Can you work these out from the drawing? Everything is in mm from the part's minimum corner. A direction names the side the tool comes from. Give positions to 0.01 mm unless a question says otherwise; leave off trailing zeros. Loops run counter-clockwise (first coordinate to the right, second up) from the corner with the lowest first, then second, coordinate; pieces in that order, holes last. Notation, with made-up numbers: (53.25, 87.5) -> (107.25, 87.5) arc R21 ccw to (107.25, 117.5) -> close; hole circle Ø7 at (55, -9.75). An arc over 180 degrees is marked (long way). Return JSON: item names as keys, results as strings. Group by question number.
Q1. I need wall thicknesses on line 1 along Z through (x, y) = (20, 0.7); line 2 along Z through (x, y) = (18, 2.4); line 3 along Y through (x, z) = (22, 28). Which ranges of each line are inside material? Lowest first, please. Write a range as [from, to].
Q2. Suppose I cut it at B-B, the plane z = 20. Please give me the cut outline in (x, y).
Q3. Will these pins go through, and if not, where does the flat tip stop? pin 1 (1.5 mm diameter, centred on y = 3.5, z = 29.5, fed in from -X) (1 decimal); pin 2 (0.6 mm diameter, centred on x = 18.5, y = 3, fed in from -Z); pin 3 (1.5 mm diameter, centred on x = 29, y = 3.5, fed in from -Z); pin 4 (2 mm diameter, centred on x = 20, z = 35, fed in from -Y).
Q4. Which directions (+Z, -Z, +X, -X, +Y, -Y) give clear straight access to the entire face, cutting with the end or side of a thin tool? Please do the marked faces 1, 2, 3 and 4.
Q5. Thinking about a two-plate mould opening in Z: for the marked faces 5, 6 and 7, which applies, pulls with the +Z half, pulls with the -Z half, needs draft (parallel to the pull), parting line crosses it, or undercut?
Q6. Suppose I cut it at C-C, the plane x = 20. Please give me the cut outline in (y, z).
Q7. Suppose I cut it at A-A, the plane y = 1.2. Please give me the cut outline in (x, z), and give its area (3 significant figures).
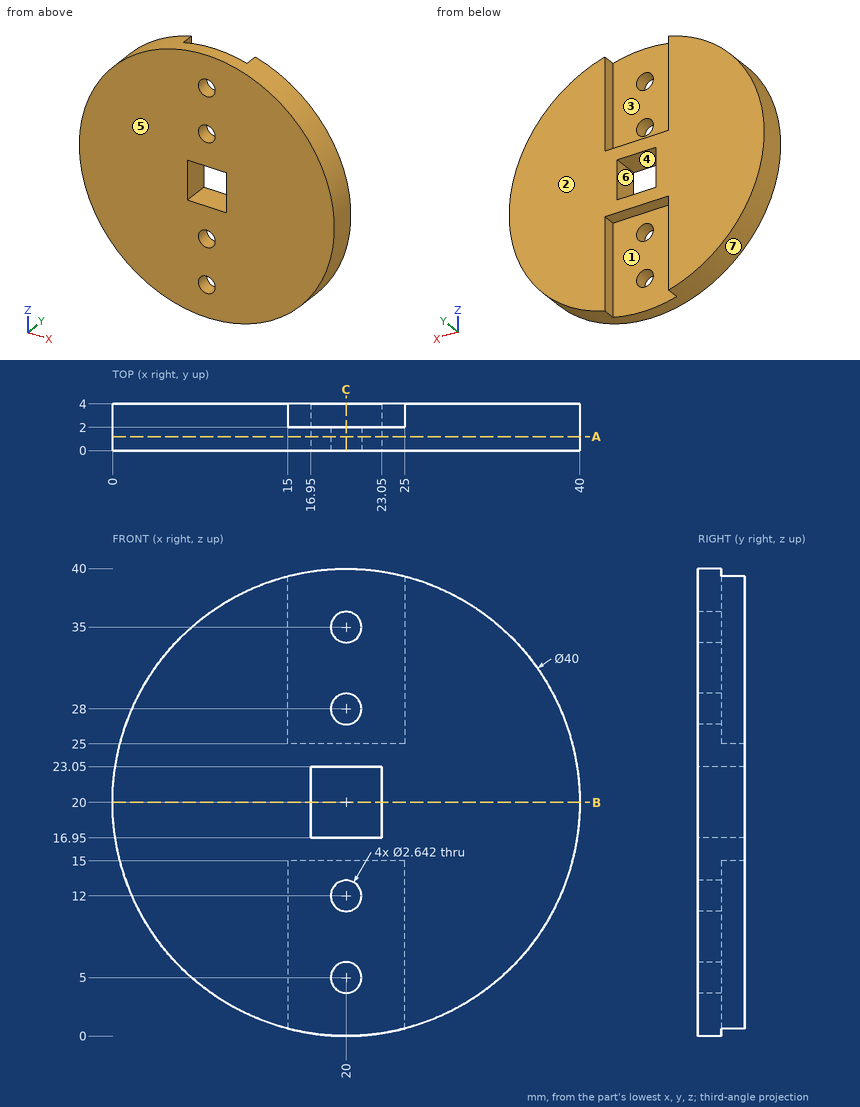
Ans:
{
 "1": {"line 1": "z = [0, 3.68], [6.32, 10.68], [13.32, 16.95], [23.05, 26.68], [29.32, 33.68], [36.32, 40]", "line 2": "z = [15, 16.95], [23.05, 25]", "line 3": "y = [0, 2]"},
 "2": {"outline": "(0, 0) -> (16.95, 0) -> (16.95, 4) -> (0, 4) -> close; (23.05, 0) -> (40, 0) -> (40, 4) -> (23.05, 4) -> close"},
 "3": {"pin 1": "stops at x = 2", "pin 2": "stops at z = 15", "pin 3": "stops at z = 1.78", "pin 4": "passes through"},
 "4": {"face 1": "-Z, +Y", "face 2": "+Z, -Z, +X, -X, +Y", "face 3": "+Z, +Y", "face 4": "+Y, -Y"},
 "5": {"face 5": "needs draft", "face 6": "undercut", "face 7": "parting line crosses it"},
 "6": {"outline": "(0, 0) -> (2, 0) -> (2, 3.68) -> (0, 3.68) -> close; (0, 6.32) -> (2, 6.32) -> (2, 10.68) -> (0, 10.68) -> close; (0, 13.32) -> (2, 13.32) -> (2, 15) -> (4, 15) -> (4, 16.95) -> (0, 16.95) -> close; (0, 23.05) -> (4, 23.05) -> (4, 25) -> (2, 25) -> (2, 26.68) -> (0, 26.68) -> close; (0, 29.32) -> (2, 29.32) -> (2, 33.68) -> (0, 33.68) -> close; (0, 36.32) -> (2, 36.32) -> (2, 40) -> (0, 40) -> close"},
 "7": {"outline": "circle Ø40 at (20, 20); hole (16.95, 16.95) -> (23.05, 16.95) -> (23.05, 23.05) -> (16.95, 23.05) -> close; hole circle Ø2.64 at (20, 5); hole circle Ø2.64 at (20, 12); hole circle Ø2.64 at (20, 28); hole circle Ø2.64 at (20, 35)", "area": "1,200 mm^2"}
}
